Check sheet for the modelled part. Datum: model origin and axes. Units: mm. A direction names the side the tool comes from. Give positions to 0.01 mm unless a question says otherwise; leave off trailing zeros. Order: outer loops, then holes, each group sorted by start corner. A loop starts at its lowest first (then second) coordinate and runs counter-clockwise, first axis right, second up. Notation, with made-up numbers: (-38, 22.25) -> (-14, 22.25) arc R17 ccw to (-14, 40.25) -> close; hole circle Ø5 at (38.5, 9.5). An arc over 180 degrees is marked (long way). Write each question's results on one line, items separated by ' | '.
from build123d import *

# Parameters (mm, degrees)
F0_R     = 2.476830384
F0_W     = 1.4847664508
F0_H     = 6.35
F1_DEPTH = 10.16
F2_R     = 2.54


with BuildPart() as f1:
    # F0 (on Right) → F1 (new body)
    with BuildSketch(Plane.YZ):
        Polygon((-12.7859174941, 41.275), (-25.4859174941, 41.275), (-25.4859174941, 0), (-12.7859174941, 18.1374796856), align=None)
        Polygon((-12.7859174941, 18.1374796856), (-25.4859174941, 0), (-12.7859174941, -18.1374796856), (-12.7859174941, 0), align=None)
        with BuildLine():
            Line((-12.7859174941, 0), (-12.7859174941, -18.1374796856))
            Line((-12.7859174941, -18.1374796856), (-3.8262820868, -30.9331651338))
            ThreePointArc((-3.8262820868, -30.9331651338), (-4.9808453905, -22.1615497886), (-1.7649908775, -13.9194304048))
            Line((-1.7649908775, -13.9194304048), (-12.7859174941, 0))
        make_face()
        Polygon((-12.7859174941, -18.1374796856), (-25.4859174941, 0), (-25.4859174941, -41.275), (-12.7859174941, -41.275), align=None)
        with BuildLine():
            ThreePointArc((-1.7649908775, -13.9194304048), (-4.9808453905, -22.1615497886), (-3.8262820868, -30.9331651338))
            Line((-3.8262820868, -30.9331651338), (0.7948947361, -37.5328896022))
            ThreePointArc((0.7948947361, -37.5328896022), (4.4509166454, -40.0662604083), (8.6213238247, -41.6129238499))
            Line((8.6213238247, -41.6129238499), (16.7188414486, -41.6129238499))
            ThreePointArc((16.7188414486, -41.6129238499), (18.1090826399, -41.2277000329), (19.4635172648, -40.731036358))
            Line((19.4635172648, -40.731036358), (12.2868024965, -31.6668455484))
            ThreePointArc((12.2868024965, -31.6668455484), (6.8866357903, -28.8791743085), (5.4117238908, -22.9836212144))
            Line((5.4117238908, -22.9836212144), (-1.7649908775, -13.9194304048))
        make_face()
        with BuildLine():
            ThreePointArc((30.4500826367, -24.300039859), (18.1231915168, -7.3769194747), (-1.7649908775, -13.9194304048))
            Line((-1.7649908775, -13.9194304048), (5.4117238908, -22.9836212144))
            ThreePointArc((5.4117238908, -22.9836212144), (13.3309493362, -16.9529326094), (20.0468522367, -24.300039859))
            ThreePointArc((20.0468522367, -24.300039859), (17.7489289843, -29.6499977568), (12.2868024965, -31.6668455484))
            Line((12.2868024965, -31.6668455484), (19.4635172648, -40.731036358))
            ThreePointArc((19.4635172648, -40.731036358), (27.4504017754, -34.182881867), (30.4500826367, -24.300039859))
        make_face()
        with BuildLine():
            Line((-1.5775528515, 34.1446833088), (-12.7859174941, 18.1374796856))
            Line((-12.7859174941, 18.1374796856), (-12.7859174941, 0))
            Line((-12.7859174941, 0), (2.9841893191, 19.9176450311))
            ThreePointArc((2.9841893191, 19.9176450311), (-1.763802881, 26.2401091232), (-1.5775528515, 34.1446833088))
        make_face()
        with BuildLine():
            Line((17.9186733985, 38.7798985425), (2.9841893191, 19.9176450311))
            ThreePointArc((2.9841893191, 19.9176450311), (12.2603418149, 18.1282692763), (19.9820541252, 23.5710654062))
            Line((19.9820541252, 23.5710654062), (19.9820541252, 36.2767071198))
            ThreePointArc((19.9820541252, 36.2767071198), (19.0348785601, 37.5979683806), (17.9186733985, 38.7798985425))
        make_face()
        with BuildLine():
            Line((1.8930880599, 39.1012722086), (-1.5775528515, 34.1446833088))
            ThreePointArc((-1.5775528515, 34.1446833088), (-1.763802881, 26.2401091232), (2.9841893191, 19.9176450311))
            Line((2.9841893191, 19.9176450311), (17.9186733985, 38.7798985425))
            ThreePointArc((17.9186733985, 38.7798985425), (15.4927249878, 40.5209748262), (12.7134769516, 41.6129238499))
            Line((12.7134769516, 41.6129238499), (6.7366465898, 41.6129238499))
            ThreePointArc((6.7366465898, 41.6129238499), (4.171026982, 40.6344848722), (1.8930880599, 39.1012722086))
        make_face()
        with Locations((3.3962282663, 29.923886263)):
            Circle(F0_R, mode=Mode.SUBTRACT)
        Polygon((23.5980694161, 39.3109042168), (19.9820541252, 36.2767071198), (23.5980694161, 36.2767071198), align=None)
        with BuildLine():
            ThreePointArc((21.7900617707, 29.923886263), (21.3292601006, 26.6213408627), (19.9820541252, 23.5710654062))
            Line((19.9820541252, 23.5710654062), (23.5980694161, 23.5710654062))
            Line((23.5980694161, 23.5710654062), (23.5980694161, 25.4382899789))
            Line((23.5980694161, 25.4382899789), (22.1133029653, 26.748886263))
            Line((22.1133029653, 26.748886263), (22.1133029653, 33.098886263))
            Line((22.1133029653, 33.098886263), (23.5980694161, 33.098886263))
            Line((23.5980694161, 33.098886263), (23.5980694161, 36.2767071198))
            Line((23.5980694161, 36.2767071198), (19.9820541252, 36.2767071198))
            ThreePointArc((19.9820541252, 36.2767071198), (21.3292601006, 33.2264316634), (21.7900617707, 29.923886263))
        make_face()
        with BuildLine():
            Line((19.9820541252, 36.2767071198), (19.9820541252, 23.5710654062))
            ThreePointArc((19.9820541252, 23.5710654062), (21.3292601006, 26.6213408627), (21.7900617707, 29.923886263))
            ThreePointArc((21.7900617707, 29.923886263), (21.3292601006, 33.2264316634), (19.9820541252, 36.2767071198))
        make_face()
        with Locations((22.8556861907, 29.923886263)):
            Rectangle(F0_W, F0_H)
        Polygon((22.1133029653, 26.748886263), (23.5980694161, 25.4382899789), (23.5980694161, 26.748886263), align=None)
        Polygon((23.5980694161, 23.5710654062), (19.9820541252, 23.5710654062), (23.5980694161, 20.5368683093), align=None)
        Polygon((44.9733029653, 33.098886263), (23.5980694161, 33.098886263), (23.5980694161, 26.748886263), (40.9346896774, 26.748886263), (44.9733029653, 26.748886263), align=None)
        Polygon((23.5980694161, 26.748886263), (23.5980694161, 25.4382899789), (24.8001961815, 24.3771784008), (27.4288224834, 25.4811998457), (31.844913851, 22.8000022471), (34.2106743562, 25.3234822303), (35.9455681252, 24.3771784008), (39.1914657905, 24.3771784008), (40.9346896774, 26.748886263), align=None)
        Polygon((48.0538682116, 29.7363082874), (44.9733029653, 33.098886263), (44.9733029653, 26.748886263), (40.9346896774, 26.748886263), (43.0080477987, 22.1112590571), align=None)
    extrude(amount=F1_DEPTH)

    # F2
    f2_edges = [f1.edges().sort_by_distance(p)[0] for p in [
        (10.16, -25.485917, 0),
        (10.16, -19.135917, 41.275),
        (5.08, -12.785917, 41.275),
        (0, -19.135917, 41.275),
        (5.08, -25.485917, 41.275),
        (0, -25.485917, 0),
        (10.16, -5.446415, 28.619376),
        (10.16, -12.785917, 29.70624),
        (10.16, -4.900864, 9.958823),
        (0, -4.900864, 9.958823),
        (10.16, -7.275454, -6.959715),
        (0, -7.275454, -6.959715),
        (10.16, -12.785917, -29.70624),
        (0, -12.785917, -29.70624),
        (0, -19.135917, -41.275),
        (5.08, -12.785917, -41.275),
        (10.16, -19.135917, -41.275),
        (5.08, -25.485917, -41.275),
        (5.08, 12.713477, 41.612924),
        (10.16, -5.995511, -27.835185),
        (0, -5.995511, -27.835185),
    ]]
    fillet(f2_edges, radius=F2_R)


solid = f1.part
1. Access from +Z, -Z, +X, -X, +Y, -Y to the whole of each face (thin tool, end or side, straight path). Record for faces 1 (the flat face through (5, -19, -41.275)), 2 (the flat face through (5, 21.8, 37.8)), 3 (the cylindrical face through (9.396, -19.189, 40.551)), 4 (the cylindrical face through (0.764, -19.083, -40.551)).
Verdict:
face 1: -Z, +X, -X, -Y | face 2: +Z, +X, -X | face 3: +Z, +X, -Y | face 4: -Z, -X, -Y
2. Mould release check, pull along Z, two halves, no side actions. Record for faces 5 (the cylindrical face through (9.4, -8.27, -6.88)), 6 (the cylindrical face through (5.009, 4.205, 40.652)), 7 (the cylindrical face through (0.764, -5.951, 9.799)), 8 (the cylindrical face through (5.12, -13.55, -40.55)): +Z half, -Z half, draft (parallel to the pull), parting line (faces both ways), or undercut.
Verdict:
face 5: undercut | face 6: +Z half | face 7: undercut | face 8: -Z half
3. Gauge pin test, flat ends, axial feed: pin 1 Ø1.9 at (x, z) = (7, 37) entering from +Y; pin 2 Ø1 at (x, z) = (8, -19) entering from +Y; pin 3 Ø2.5 at (x, z) = (5, -25) entering from +Y. Record the tip position at first contact, or that the pin passes through.
Verdict:
pin 1: stops at y = 23.6 | pin 2: stops at y = 29.79 | pin 3: stops at y = 30.45
4. Section check D-D on y = 38. Record the cut outline in (x, z), then the cut area to 3 significant figures.
Verdict:
outline: (0, 24.38) -> (10.16, 24.38) -> (10.16, 33.1) -> (0, 33.1) -> close | area: 88.6 mm^2
5. Material ranges on probe 1 along Z at (x, y) = (2.25, 12); probe 2 along Y at (x, z) = (9.75, 22.5); probe 3 along Z at (x, y) = (7.5, 19), recorded low to high. Write a range as from..to.
Verdict:
probe 1: z = -41.61..-31.65, -16.95..-6.53, 18.08..41.61 | probe 2: y = -24.33..-13.94, -8.32..19.24, 21.26..23.6, 42.83..43.27 | probe 3: z = -40.92..-28.09, -20.51..-7.68, 22.21..37.64
6. Section check B-B on z = -26. Give the number of separate pieces and of enclosed holes in the cut face, then the cut area to 3 significant figures.
Verdict:
separate pieces: 3 | enclosed holes: 0 | area: 357 mm^2
7. Section check A-A on y = 26. Record the cut outline in (x, z), then the cut area to 3 significant figures.
Verdict:
outline: (0, -36.07) -> (10.16, -36.07) -> (10.16, -12.53) -> (0, -12.53) -> close; (0, 24.88) -> (10.16, 24.88) -> (10.16, 33.1) -> (0, 33.1) -> close | area: 323 mm^2
